Part model, mm, in its own coordinate system. Face numbers are marked on the shaded views. Round coordinates to 2 decimals unless told otherwise and drop trailing zeros. Use a Markdown table: item, result. Add a question column.
1) Two-plate mould, pull along Z, no slides. Class the marked faces 1, 2 and 3: released by +Z, released by -Z, zero draft, split by the parting line, or undercut.
2) Drop flat-ended pins along their axis: P1, Ø1, axis at y = 131, z = 57.5, coming from the +X side; P2, Ø5, axis at y = 142, z = 52, coming from the -X side; P3, Ø10, axis at y = 111, z = 122, coming from the +X side. Give the stop position or say it passes through.
3) Wall check: probe 1 along Z at (x, y) = (0, 110.5); probe 2 along Z at (x, y) = (0, 140); probe 3 along X at (y, z) = (116, 145.5). Give the ranges that are in metal, low to high.
```python
from build123d import *

# Parameters (mm, degrees)
BOSS_EXTRUDE1_DEPTH     = 300
SKETCH3_R               = 15.5
CUT_EXTRUDE1_DEPTH      = 23
CUT_EXTRUDE1_DEPTH_BACK = 23
SKETCH4_R               = 35
CUT_EXTRUDE3_DEPTH      = 300
SKETCH5_W               = 488.913893014
SKETCH5_H               = 228.614771509
SKETCH5_W_2             = 496.713117629
SKETCH5_H_2             = 107.726789986
CUT_EXTRUDE4_DEPTH      = 201.0000001


with BuildPart() as part:
    # Sketch1 → Boss-Extrude1 (new body)
    with BuildSketch(Plane(origin=(0, 0, 0), x_dir=(1, 0, 0), z_dir=(0, 1, 0))):
        with BuildLine():
            Line((-200, 1e-09), (200, 1e-09))
            add(Edge.make_bspline(
                [(-200, 1e-09), (0, -400.000000001), (200, 1e-09)],
                knots=[0.056028396, 0.056028396, 0.056028396, 0.943971604, 0.943971604, 0.943971604], degree=2))
        make_face()
    extrude(amount=BOSS_EXTRUDE1_DEPTH)

    # Sketch3 → Cut-Extrude1 (cut, two sides)
    with BuildSketch(Plane(origin=(0, 150, 0), x_dir=(1, 0, 0), z_dir=(0, 1, 0))) as cut_extrude1_sk:
        with Locations((0, -142.999999999)):
            Circle(SKETCH3_R)
    extrude(amount=CUT_EXTRUDE1_DEPTH, mode=Mode.SUBTRACT)
    extrude(cut_extrude1_sk.sketch, amount=-CUT_EXTRUDE1_DEPTH_BACK, mode=Mode.SUBTRACT)

    # Sketch4 → Cut-Extrude3 (cut)
    with BuildSketch(Plane(origin=(0, 173, 0), x_dir=(1, 0, 0), z_dir=(0, 1, 0))):
        with Locations((0, -142.999999999)):
            Circle(SKETCH4_R)
    cut_extrude3 = extrude(amount=CUT_EXTRUDE3_DEPTH, mode=Mode.SUBTRACT)

    # Mirror1: Cut-Extrude3 across plane
    add(cut_extrude3.mirror(Plane.ZX.offset(150)), mode=Mode.SUBTRACT)

    # Sketch5 → Cut-Extrude4 (cut, through all)
    with BuildSketch(Plane(origin=(0, 0, 0), x_dir=(-1, 0, 0), z_dir=(0, 0, -1))):
        with Locations((-0.974903077, 261.907385755)):
            Rectangle(SKETCH5_W, SKETCH5_H)
        with Locations((2.92470923, 42.936605007)):
            Rectangle(SKETCH5_W_2, SKETCH5_H_2)
    extrude(amount=-CUT_EXTRUDE4_DEPTH, mode=Mode.SUBTRACT)


solid = part.part
```
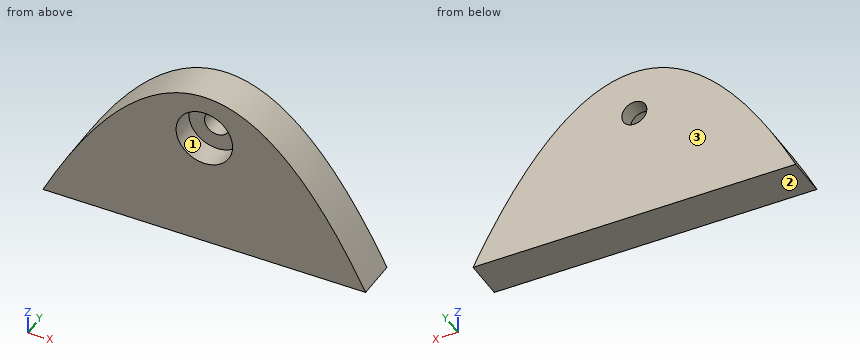
Entries:
| question | item | result |
|---|---|---|
| 1 | face 1 | undercut |
| 1 | face 2 | released by -Z |
| 1 | face 3 | zero draft |
| 2 | P1 | stops at x = 169.12 |
| 2 | P2 | stops at x = -173.49 |
| 2 | P3 | stops at x = 128.84 |
| 3 | probe 1 | z = 0 to 108, 178 to 200 |
| 3 | probe 2 | z = 0 to 127.5, 158.5 to 200 |
| 3 | probe 3 | x = -104.4 to -34.91, 34.91 to 104.4 |
